from build123d import *

# Parameters (mm, degrees)
F1_DEPTH        = 177.8
F3_DEPTH        = 9.906
F4_W            = 4.572
F4_H            = 177.8
F5_DEPTH        = 10.16
F7_DEPTH        = 35.56
F9_D            = 8.89
F9_DEPTH        = 5.08
F9_TIP          = 2.6708254516
F10_D           = 6.35
F10_CBORE_D     = 16.51
F10_CBORE_DEPTH = 35.56
F11_T1_DEPTH    = 184.3320747894
F11_T3_DEPTH    = 52.2520747894
F11_T5_DEPTH    = 181.6882193011


# Not quite as in the source:
# - a fillet or chamfer that OpenCascade refuses, or shapes differently, is made with other operations: its cross-section is extruded or revolved along the edge and cut away or added


with BuildPart() as f1:
    # F0 (on Front) → F1 (new body)
    with BuildSketch(Plane.XZ):
        Polygon((0, 44.45), (0, 0), (31.75, 0), (31.75, 19.05), (34.29, 19.05), (34.29, 0), (44.45, 0), (44.45, 25.4), (33.4514773719, 44.45), align=None)
    extrude(amount=F1_DEPTH)

    # F2 (on face) → F3 (cut)
    with BuildSketch(Plane(origin=(0, 0, 0), x_dir=(0, -1, 0), z_dir=(-1, 0, 0))):
        with BuildLine():
            Line((177.8, 20.828), (177.8, 44.45))
            Line((177.8, 44.45), (45.72, 44.45))
            Line((45.72, 44.45), (45.72, 27.178))
            ThreePointArc((45.72, 27.178), (47.5798719395, 22.6878719395), (52.07, 20.828))
            Line((52.07, 20.828), (177.8, 20.828))
        make_face()
    extrude(amount=-F3_DEPTH, mode=Mode.SUBTRACT)

    # F4 (on face) → F5 (cut)
    with BuildSketch(Plane.XY.offset(44.45)):
        with Locations((9.906, -88.9)):
            Rectangle(F4_W, F4_H)
    extrude(amount=-F5_DEPTH, mode=Mode.SUBTRACT)

    # F6 (on face) → F7 (cut)
    with BuildSketch(Plane.XY.offset(44.45)):
        with BuildLine():
            Line((7.62, -177.8), (12.192, -177.8))
            Line((12.192, -177.8), (12.192, -45.72))
            ThreePointArc((12.192, -45.72), (9.906, -43.434), (7.62, -45.72))
            Line((7.62, -45.72), (7.62, -177.8))
        make_face()
    extrude(amount=-F7_DEPTH, mode=Mode.SUBTRACT)

    # F9
    with Locations(Plane(origin=(0, 0, 0), x_dir=(1, 0, 0), z_dir=(0, 0, -1))):
        with Locations((26.67, 38.1)):
            Hole(F9_D / 2, depth=F9_DEPTH)
            with Locations((0, 0, -(F9_DEPTH + F9_TIP / 2))):  # 118° drill point
                Cone(0, F9_D / 2, F9_TIP, mode=Mode.SUBTRACT)

    # F10 (through all)
    with Locations(Plane(origin=(0, 0, 0), x_dir=(1, 0, 0), z_dir=(0, 0, -1))):
        with Locations((22.86, 25.4)):
            CounterBoreHole(F10_D / 2, F10_CBORE_D / 2, F10_CBORE_DEPTH)

    # F11: chamfer of 1.27 on 6 edges, made by hand

    # F11_s2 → F11_t1 (cut)
    with BuildSketch(Plane.XZ.offset(-3.2660373947)):
        Polygon((12.192, 43.18), (13.462, 44.45), (12.192, 44.45), align=None)
        Polygon((0, 1.27), (1.27, 0), (0, 0), align=None)
        Polygon((44.45, 1.27), (43.18, 0), (44.45, 0), align=None)
    extrude(amount=F11_T1_DEPTH, mode=Mode.SUBTRACT)

    # F11_s4 → F11_t3 (cut)
    with BuildSketch(Plane.XZ.offset(-3.2660373947)):
        Polygon((6.35, 44.45), (7.62, 43.18), (7.62, 44.45), align=None)
        Polygon((0, 43.18), (1.27, 44.45), (0, 44.45), align=None)
    extrude(amount=F11_T3_DEPTH, mode=Mode.SUBTRACT)

    # F11_s6 → F11_t5 (cut)
    with BuildSketch(Plane.XZ.offset(-1.9441096505)):
        Polygon((32.7182425301, 44.45), (33.8180947929, 43.815), (33.4514773719, 44.45), align=None)
    extrude(amount=F11_T5_DEPTH, mode=Mode.SUBTRACT)


solid = f1.part
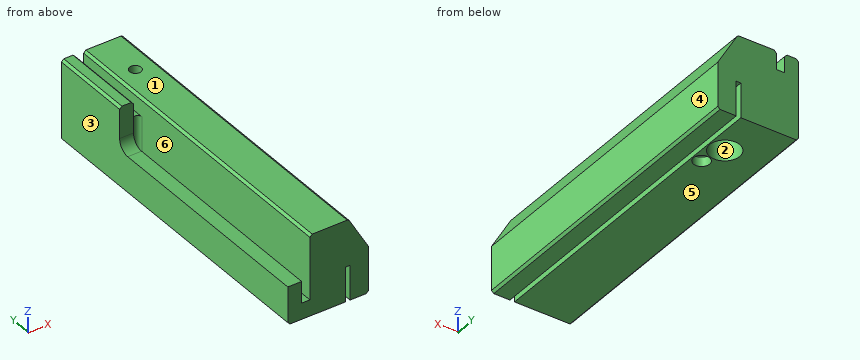
The listing builds one solid part. Answer for the finished solid, in the listing's coordinates (mm). Face numbers are marked on the shaded views. A direction names the side the tool comes from. Give positions to 0.01 mm unless a question says otherwise; leave off trailing zeros. Loops run counter-clockwise (first coordinate to the right, second up) from the corner with the lowest first, then second, coordinate; pieces in that order, holes last. Notation, with made-up numbers: (12.25, 89) - (43.25, 89) arc R9 cw to (43.25, 104) - close; hole circle Ø8 at (76, 67). An arc over 180 degrees is marked (long way). Use one line per item in the form item = value.
1. Section C-C on y = -137.5 is taken. Give the vertices of the cut face in (x, z) (3 decimals).
Calculated:
outline = (0, 1.27) - (1.27, 0) - (31.75, 0) - (31.75, 19.05) - (34.29, 19.05) - (34.29, 0) - (43.18, 0) - (44.45, 1.27) - (44.45, 25.4) - (33.818, 43.815) - (32.718, 44.45) - (13.462, 44.45) - (12.192, 43.18) - (12.192, 8.89) - (7.62, 8.89) - (7.62, 20.828) - (0, 20.828) - close
2. Section B-B on z = 32.5 is taken. Give the vertices of the cut face in (x, y) (3 decimals).
Calculated:
outline = (0, -45.72) - (7.62, -45.72) arc R2.286 cw to (12.192, -45.72) - (12.192, -177.8) - (40.351, -177.8) - (40.351, 0) - (0, 0) - close; hole circle Ø16.51 at (22.86, -25.4)
3. The mould has two halves that part along X. Classify the marked faces 1, 2, 3 and 4: pulls with the +X half, pulls with the -X half, needs draft (parallel to the pull), parting line crosses it, or undercut.
Calculated:
face_1 = needs draft
face_2 = undercut
face_3 = pulls with the -X half
face_4 = pulls with the +X half
4. Given pin 1 Ø4 at (x, y) = (34, -133) entering from +Z; pin 2 Ø2 at (x, y) = (9.5, -36.5) entering from +Z; pin 3 Ø1.3 at (x, y) = (33.5, -67) entering from -Z; pin 4 Ø13 at (x, y) = (22.86, -25.4) entering from -Z, each flat-ended and moving along its own axis, determine where each tip first touches the part or whether it passes through.
Calculated:
pin_1 = 44.45
pin_2 = 34.29
pin_3 = 19.05
pin_4 = 35.56
5. Section D-D on x = 37 is taken. Give the vertices of the cut face in (y, z).
Calculated:
outline = (-177.8, 0) - (0, 0) - (0, 38.3) - (-177.8, 38.3) - close
6. Section A-A on y = -25.4 is taken. Give the vertices of the cut face in (x, z) (3 decimals), then the cut area to 3 significant figures.
Calculated:
outline = (0, 1.27) - (1.27, 0) - (14.605, 0) - (14.605, 35.56) - (19.685, 35.56) - (19.685, 44.45) - (13.462, 44.45) - (12.192, 43.18) - (12.192, 34.29) - (7.62, 34.29) - (7.62, 43.18) - (6.35, 44.45) - (1.27, 44.45) - (0, 43.18) - close; (26.035, 35.56) - (31.115, 35.56) - (31.115, 0) - (31.75, 0) - (31.75, 19.05) - (34.29, 19.05) - (34.29, 0) - (43.18, 0) - (44.45, 1.27) - (44.45, 25.4) - (33.818, 43.815) - (32.718, 44.45) - (26.035, 44.45) - close
area = 1,130 mm^2
7. Which of the six approach directions +Z, -Z, +X, -X, +Y, -Y give full straight-line access (tool end or side, diameter ignored) to the marked faces 5 and 6?
Calculated:
face_5 = -Z, +X, -X, +Y, -Y
face_6 = +Z, -Y
8. Find the intervals of material crossed by line 1 along X through (y, z) = (-38.1, 1.4) (3 decimals); line 2 along X through (y, z) = (-93, 10.5); line 3 along Y through (x, z) = (22.86, 38.75) (3 decimals), in increasing order. Write a range as [from, to].
Calculated:
line_1 = [0, 22.225], [31.115, 31.75], [34.29, 44.45]
line_2 = [0, 7.62], [12.19, 31.75], [34.29, 44.45]
line_3 = [-177.8, -28.575], [-22.225, 0]
